from build123d import *

# Parameters (mm, degrees)
F0_W     = 80
F0_H     = 32
F0_W_2   = 76
F0_H_2   = 28
F1_DEPTH = 52
F0_W_3   = 72
F0_H_3   = 24
F2_DEPTH = 57
F3_DEPTH = 52
F4_R     = 4
F4_W     = 11.847522
F4_H     = 22
F5_DEPTH = 47


with BuildPart() as f1:
    # F0 (on Top) → F1 (new body)
    with BuildSketch(Plane.XY):
        with Locations((-13.381271, 0.573133)):
            Rectangle(F0_W, F0_H)
        with Locations((-13.381271, 0.573133)):
            Rectangle(F0_W_2, F0_H_2, mode=Mode.SUBTRACT)
    extrude(amount=F1_DEPTH)

    # F0 (on Top) → F2 (join)
    with BuildSketch(Plane.XY):
        with Locations((-13.381271, 0.573133)):
            Rectangle(F0_W_2, F0_H_2)
        with Locations((-13.381271, 0.573133)):
            Rectangle(F0_W_3, F0_H_3, mode=Mode.SUBTRACT)
    extrude(amount=F2_DEPTH)

    # F0 (on Top) → F3 (join)
    with BuildSketch(Plane.XY):
        with Locations((-13.381271, 0.573133)):
            Rectangle(F0_W_3, F0_H_3)
    extrude(amount=F3_DEPTH)

    # F4 (on face) → F5 (cut)
    with BuildSketch(Plane.XY.offset(52)):
        with Locations((-42.881271, -4.926867)):
            Circle(F4_R)
        with Locations((-34.529625, 0.573133)):
            Circle(F4_R)
        with Locations((-26.177978, -4.926867)):
            Circle(F4_R)
        with Locations((-26.177978, 6.073133)):
            Circle(F4_R)
        with Locations((-42.881271, 6.073133)):
            Circle(F4_R)
        with Locations((14.454672, 0.753674)):
            Rectangle(F4_W, F4_H)
    extrude(amount=-F5_DEPTH, mode=Mode.SUBTRACT)


solid = f1.part
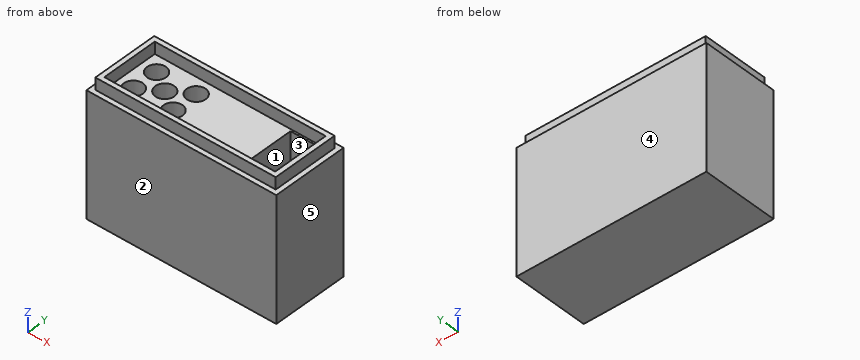
Verification items for the finished model (mm, model axes). Face numbers are marked on the shaded views. A direction names the side the tool comes from. Coordinates: 2 decimals unless noted, no trailing zeros. Order: outer loops, then holes, each group sorted by start corner. A loop starts at its lowest first (then second) coordinate and runs counter-clockwise, first axis right, second up.
1. Sectioned sample at D-D, the plane x = -18. Record the cut outline in (y, z), and give its area (3 significant figures).
Results found:
outline: (-15.43, 0) - (16.57, 0) - (16.57, 52) - (14.57, 52) - (14.57, 57) - (12.57, 57) - (12.57, 52) - (-11.43, 52) - (-11.43, 57) - (-13.43, 57) - (-13.43, 52) - (-15.43, 52) - close
area: 1,680 mm2
2. Sectioned sample at C-C, the plane y = -2.5. Record the cut outline in (x, z), and give its area (3 significant figures).
Results found:
outline: (-53.38, 0) - (26.62, 0) - (26.62, 52) - (24.62, 52) - (24.62, 57) - (22.62, 57) - (22.62, 52) - (20.38, 52) - (20.38, 5) - (8.53, 5) - (8.53, 52) - (-23, 52) - (-23, 5) - (-29.36, 5) - (-29.36, 52) - (-31.97, 52) - (-31.97, 5) - (-37.09, 5) - (-37.09, 52) - (-39.7, 52) - (-39.7, 5) - (-46.06, 5) - (-46.06, 52) - (-49.38, 52) - (-49.38, 57) - (-51.38, 57) - (-51.38, 52) - (-53.38, 52) - close
area: 2,780 mm2
3. Release check for a two-part mould opening along X. For the marked faces 3, 4 and 5 record: +X half, -X half, draft (parallel to the pull), parting line (faces both ways), or undercut.
Results found:
face 3: undercut
face 4: draft
face 5: +X half
4. Sectioned sample at A-A, the plane x = 13.5. Record the cut outline in (y, z).
Results found:
outline: (-15.43, 0) - (16.57, 0) - (16.57, 52) - (14.57, 52) - (14.57, 57) - (12.57, 57) - (12.57, 52) - (11.75, 52) - (11.75, 5) - (-10.25, 5) - (-10.25, 52) - (-11.43, 52) - (-11.43, 57) - (-13.43, 57) - (-13.43, 52) - (-15.43, 52) - close
5. Set-up check for the marked faces 1 and 2: record each of +Z, -Z, +X, -X, +Y, -Y from which the full face is reachable in a straight line by a thin tool's end or side.
Results found:
face 1: +Z
face 2: +Z, -Z, +X, -X, -Y
6. Go/stop test with flat-tipped pins: pin 1 Ø5 at (x, y) = (-7, 0) entering from -Z; pin 2 Ø4 at (x, y) = (15, 2.5) entering from +Z; pin 3 Ø2.5 at (x, z) = (2.5, 54) entering from +Y; pin 4 Ø5.5 at (y, z) = (-4.5, 55.5) entering from +X. Record where each tip stops, or that it passes through.
Results found:
pin 1: stops at z = 0
pin 2: stops at z = 5
pin 3: stops at y = 14.57
pin 4: stops at x = 24.62
7. Sectioned sample at B-B, the plane z = 32.5. Record the cut outline in (x, y), and give its area (3 significant figures).
Results found:
outline: (-53.38, -15.43) - (26.62, -15.43) - (26.62, 16.57) - (-53.38, 16.57) - close; hole circle Ø8 at (-42.88, -4.93); hole circle Ø8 at (-42.88, 6.07); hole circle Ø8 at (-34.53, 0.57); hole circle Ø8 at (-26.18, -4.93); hole circle Ø8 at (-26.18, 6.07); hole (8.53, -10.25) - (20.38, -10.25) - (20.38, 11.75) - (8.53, 11.75) - close
area: 2,050 mm2
8. Scan lines: line 1 (X direction, y = 6, z = 29.5); line 2 (X direction, y = -7.5, z = 41); line 3 (Y direction, x = -40, z = 29.5). Record each from-to range of solid material in increasing order.
Results found:
line 1: x = -53.38 to -46.88, -38.88 to -30.18, -22.18 to 8.53, 20.38 to 26.62
line 2: x = -53.38 to -45.94, -39.82 to -29.24, -23.12 to 8.53, 20.38 to 26.62
line 3: y = -15.43 to -7.7, -2.15 to 3.3, 8.85 to 16.57
